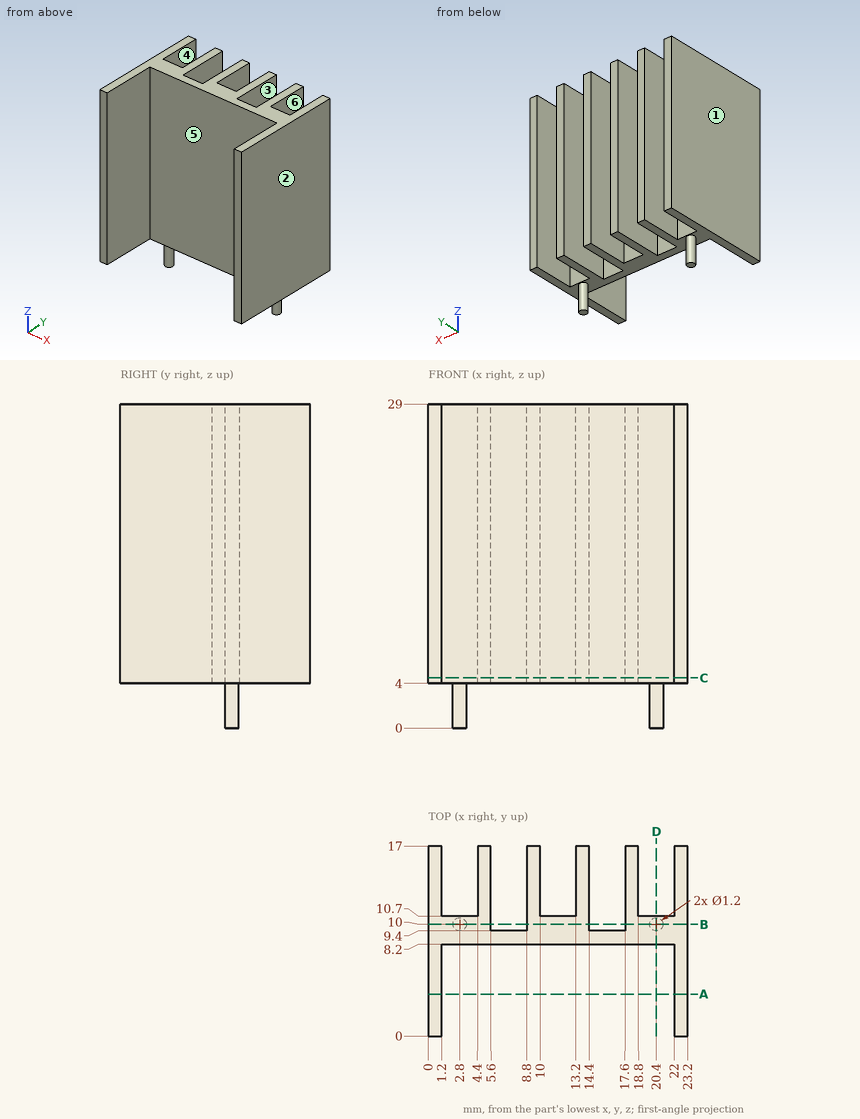
Print and shaded views of the part. All mm, measured from the part's lowest x, y and z. A direction names the side the tool comes from. Give positions to 0.01 mm unless a question says otherwise; leave off trailing zeros. Loops run counter-clockwise (first coordinate to the right, second up) from the corner with the lowest first, then second, coordinate; pieces in that order, holes last. Notation, with made-up numbers: (-15, 39.5) - (28, 39.5) arc R8 cw to (28, 49.5) - close; hole circle Ø8 at (70.25, 67.25). An arc over 180 degrees is marked (long way). One line per item, written item: value. Start each with the question number.
1. Probe L1, parallel to X at y = 11.25, z = 7.25; L2, parallel to X at y = 10, z = 20; L3, parallel to X at y = 6.5, z = 9. List the from-to ranges inside material, lowest first. Write a range as from..to.
2. Slice it at A-A (y = 3.75). List the corners of the cut face in (x, z), plus the area to 3 significant figures.
3. Slice it at D-D (x = 20.4). List the corners of the cut face in (y, z), plus the area to 3 significant figures.
4. Slice it at C-C (z = 4.5). List the corners of the cut face in (x, y), plus the area to 3 significant figures.
5. Slice it at B-B (y = 10). List the corners of the cut face in (x, z).
6. Which spindle directions (+Z, -Z, +X, -X, +Y, -Y) get a long thin tool onto all of the face, cutting with end or side? Do the marked faces 5 and 6. Say none if no direction does.
7. Pin check, flat tips, straight feed: pin 1 (4 mm diameter, centred on x = 17.5, z = 24.5, fed in from -Y); pin 2 (1.6 mm diameter, centred on x = 7, z = 19, fed in from +Y); pin 3 (4 mm diameter, centred on x = 12.5, y = 13, fed in from -Z). Stop position of each tip, or through.
8. Pull direction X, two halves, no side cores. Call the marked faces 1, 2, 3 and 4: pulls with the +X half, pulls with the -X half, needs draft (parallel to the pull), parting line crosses it, or undercut.
Solution:
1. L1: x = 0..1.2, 4.4..5.6, 8.8..10, 13.2..14.4, 17.6..18.8, 22..23.2
1. L2: x = 0..5.6, 8.8..14.4, 17.6..23.2
1. L3: x = 0..1.2, 22..23.2
2. outline: (0, 4) - (1.2, 4) - (1.2, 29) - (0, 29) - close; (22, 4) - (23.2, 4) - (23.2, 29) - (22, 29) - close
2. area: 60.0 mm^2
3. outline: (8.2, 4) - (9.4, 4) - (9.4, 0) - (10.6, 0) - (10.6, 4) - (10.7, 4) - (10.7, 29) - (8.2, 29) - close
3. area: 67.3 mm^2
4. outline: (0, 0) - (1.2, 0) - (1.2, 8.2) - (22, 8.2) - (22, 0) - (23.2, 0) - (23.2, 17) - (22, 17) - (22, 10.7) - (18.8, 10.7) - (18.8, 17) - (17.6, 17) - (17.6, 9.4) - (14.4, 9.4) - (14.4, 17) - (13.2, 17) - (13.2, 10.7) - (10, 10.7) - (10, 17) - (8.8, 17) - (8.8, 9.4) - (5.6, 9.4) - (5.6, 17) - (4.4, 17) - (4.4, 10.7) - (1.2, 10.7) - (1.2, 17) - (0, 17) - close
4. area: 115 mm^2
5. outline: (0, 4) - (2.2, 4) - (2.2, 0) - (3.4, 0) - (3.4, 4) - (5.6, 4) - (5.6, 29) - (0, 29) - close; (8.8, 4) - (14.4, 4) - (14.4, 29) - (8.8, 29) - close; (17.6, 4) - (19.8, 4) - (19.8, 0) - (21, 0) - (21, 4) - (23.2, 4) - (23.2, 29) - (17.6, 29) - close
6. face 5: +Z, -Z, -Y
6. face 6: +Z, -Z, +Y
7. pin 1: stops at y = 8.2
7. pin 2: stops at y = 9.4
7. pin 3: stops at z = 4
8. face 1: pulls with the -X half
8. face 2: pulls with the +X half
8. face 3: undercut
8. face 4: undercut
